Check sheet for the modelled part. Datum: model origin and axes. Units: mm. A direction names the side the tool comes from. Coordinates: 2 decimals unless noted, no trailing zeros. Loops run counter-clockwise (first coordinate to the right, second up) from the corner with the lowest first, then second, coordinate; pieces in that order, holes last. Notation, with made-up numbers: M 87.5,40 L 141.5,40 A27 ccw 141.5,72 Z; hole C 65,-6 d5. An arc over 180 degrees is marked long. Return JSON: item names as keys, results as strings.
from build123d import *

# Parameters (mm, degrees)
SKETCH1_R           = 30
SKETCH1_R_2         = 17.5
BOSS_EXTRUDE1_DEPTH = 9.25
SKETCH2_R           = 1.6
CUT_EXTRUDE1_DEPTH  = 9.25
CUT_EXTRUDE2_DEPTH  = 4
SKETCH4_R           = 23.5
CUT_EXTRUDE3_DEPTH  = 5.5
SKETCH5_R           = 18.5
CUT_EXTRUDE4_DEPTH  = 8.25
CIRPATTERN1_COUNT   = 6
CHAMFER1_SIZE       = 1


with BuildPart() as part:
    # Sketch1 → Boss-Extrude1 (new body)
    with BuildSketch(Plane(origin=(0, 0, 0), x_dir=(1, 0, 0), z_dir=(0, 1, 0))):
        with Locations(Location((0, 0, 0), (0, 0, 270))):
            Circle(SKETCH1_R)
        with Locations(Location((0, 0, 0), (0, 0, 270))):
            Circle(SKETCH1_R_2, mode=Mode.SUBTRACT)
    extrude(amount=BOSS_EXTRUDE1_DEPTH)

    # Sketch2 → Cut-Extrude1 (cut)
    with BuildSketch(Plane(origin=(0, 9.25, 0), x_dir=(1, 0, 0), z_dir=(0, 1, 0))):
        with Locations(Location((-27, 0, 0), (0, 0, 270))):
            Circle(SKETCH2_R)
    cut_extrude1 = extrude(amount=-CUT_EXTRUDE1_DEPTH, mode=Mode.SUBTRACT)

    # Sketch3 → Cut-Extrude2 (cut)
    with BuildSketch(Plane(origin=(0, 9.25, 0), x_dir=(1, 0, 0), z_dir=(0, 1, 0))):
        with BuildLine():
            Line((-27, 3), (-31.510174131, 3))
            Line((-31.510174131, 3), (-31.510174131, -3))
            Line((-31.510174131, -3), (-27, -3))
            ThreePointArc((-27, -3), (-24, 0), (-27, 3))
        make_face()
    cut_extrude2 = extrude(amount=-CUT_EXTRUDE2_DEPTH, mode=Mode.SUBTRACT)

    # Sketch4 → Cut-Extrude3 (cut)
    with BuildSketch(Plane.XZ):
        with Locations(Location((0, 0, 0), (0, 0, 270))):
            Circle(SKETCH4_R)
    extrude(amount=-CUT_EXTRUDE3_DEPTH, mode=Mode.SUBTRACT)

    # Sketch5 → Cut-Extrude4 (cut)
    with BuildSketch(Plane.XZ):
        with Locations(Location((0, 0, 0), (0, 0, 270))):
            Circle(SKETCH5_R)
    extrude(amount=-CUT_EXTRUDE4_DEPTH, mode=Mode.SUBTRACT)

    # CirPattern1: Cut-Extrude1, Cut-Extrude2 ×6 about axis
    cirpattern1_axis = Axis((0, 0, 0), (0, 1, 0))
    add([cut_extrude1.rotate(cirpattern1_axis, i * 360 / CIRPATTERN1_COUNT) for i in range(1, CIRPATTERN1_COUNT)], mode=Mode.SUBTRACT)
    add([cut_extrude2.rotate(cirpattern1_axis, i * 360 / CIRPATTERN1_COUNT) for i in range(1, CIRPATTERN1_COUNT)], mode=Mode.SUBTRACT)

    # Chamfer1
    chamfer1_edges = [part.edges().sort_by_distance(p)[0] for p in [
        (-25.980762114, 9.25, 15),
        (6.304127327, 9.25, 29.330154767),
        (25.980762114, 9.25, 15),
        (25.980762114, 9.25, -15),
        (0, 9.25, -30),
        (-25.980762114, 9.25, -15),
    ]]
    chamfer(chamfer1_edges, length=CHAMFER1_SIZE)


solid = part.part
1) Section check D-D on y = 7. Record the cut outline in (x, z), then the cut area to 3 significant figures.
Answers:
{"outline": "M -29.85,-3 A30 ccw -17.52,-24.35 L -16.1,-21.88 A3 cw -10.9,-24.88 L -12.33,-27.35 A30 ccw 12.33,-27.35 L 10.9,-24.88 A3 cw 16.1,-21.88 L 17.52,-24.35 A30 ccw 29.85,-3 L 27,-3 A3 cw 27,3 L 29.85,3 A30 ccw 17.52,24.35 L 16.1,21.88 A3 cw 10.9,24.88 L 12.33,27.35 A30 ccw -12.33,27.35 L -10.9,24.88 A3 cw -16.1,21.88 L -17.52,24.35 A30 ccw -29.85,3 L -27,3 A3 cw -27,-3 Z; hole C 0,0 d37", "area": "1,560 mm²"}
2) Section check C-C on y = 3.75. Record the cut outline in (x, z), then the cut area to 3 significant figures.
Answers:
{"outline": "C 0,0 d60; hole C -27,0 d3.2; hole C 0,0 d47; hole C -13.5,-23.38 d3.2; hole C -13.5,23.38 d3.2; hole C 13.5,-23.38 d3.2; hole C 13.5,23.38 d3.2; hole C 27,0 d3.2", "area": "1,040 mm²"}
3) Set-up check for faces 5 (the face through (-13.1, 5.25, 25.2)), 6 (the face through (-7.086, 6.856, -17.089)), 7 (the face through (-11.62, 7.28, 26.13)), 8 (the face through (-16.8, 7.3, 23.1)), 9 (the face through (28, 7, -3)): record each of +Z, -Z, +X, -X, +Y, -Y from which the full face is reachable in a straight line by a thin tool's end or side.
Answers:
{"face 5": "+Y", "face 6": "-Y", "face 7": "-X, +Y", "face 8": "+Z, +Y", "face 9": "+X, +Y"}
4) Draft check along Z on faces 1 (the face through (11.94, 7.28, -20.82)), 2 (the face through (-12, 9.25, -13)), 3 (the face through (16.8, 7.3, 23.1)), 4 (the face through (-25.414, 2.662, -0.208)). Enter one of: +Z half, -Z half, draft (parallel to the pull), parting line (faces both ways), or undercut.
Answers:
{"face 1": "undercut", "face 2": "draft", "face 3": "+Z half", "face 4": "undercut"}
5) Section check A-A on z = 0. Record the cut outline in (x, y).
Answers:
{"outline": "M -30,0 L -28.6,0 L -28.6,5.25 L -30,5.25 Z; M -25.4,0 L -23.5,0 L -23.5,5.5 L -18.5,5.5 L -18.5,8.25 L -17.5,8.25 L -17.5,9.25 L -24,9.25 L -24,5.25 L -25.4,5.25 Z; M 17.5,8.25 L 18.5,8.25 L 18.5,5.5 L 23.5,5.5 L 23.5,0 L 25.4,0 L 25.4,5.25 L 24,5.25 L 24,9.25 L 17.5,9.25 Z; M 28.6,0 L 30,0 L 30,5.25 L 28.6,5.25 Z"}
6) Section check B-B on x = -13.5. Record the cut outline in (y, z).
Answers:
{"outline": "M 0,-26.79 L 5.25,-26.79 L 5.25,-24.98 L 0,-24.98 Z; M 0,-21.78 L 5.25,-21.78 L 5.25,-20.38 L 9.25,-20.38 L 9.25,-11.14 L 8.25,-11.14 L 8.25,-12.65 L 5.5,-12.65 L 5.5,-19.24 L 0,-19.24 Z; M 0,19.24 L 5.5,19.24 L 5.5,12.65 L 8.25,12.65 L 8.25,11.14 L 9.25,11.14 L 9.25,20.38 L 5.25,20.38 L 5.25,21.78 L 0,21.78 Z; M 0,24.98 L 5.25,24.98 L 5.25,26.79 L 0,26.79 Z"}
7) Scan lines: line 1 along Z through (x, y) = (-13, 3.75); line 2 along X through (y, z) = (8.75, -21); line 3 along Y through (x, z) = (-16, -13.5). Record each from-to range of solid material in increasing order. Write a range as [from, to].
Answers:
{"line 1": "[-27.04, -24.9], [-21.86, -19.58], [19.58, 21.86], [24.9, 27.04]", "line 2": "[-20.72, -15.32], [-11.68, 11.68], [15.32, 20.72]", "line 3": "[5.5, 9.25]"}
8) Go/stop test with flat-tipped pins: pin 1 Ø2 at (x, z) = (15, -24.5) entering from +Y; pin 2 Ø2.5 at (x, y) = (29, 6.5) entering from +Z; pin 3 Ø3 at (y, z) = (7, -2.5) entering from -X. Record where each tip stops, or that it passes through.
Answers:
{"pin 1": "y = 5.25", "pin 2": "z = 11.4", "pin 3": "x = -29.85"}
